For this review, use the dimensioned drawing (mm, ordinates from the lowest corner) and the shaded views. Give positions to 0.01 mm unless a question says otherwise; leave off trailing zeros. Order: outer loops, then holes, each group sorted by start corner. A loop starts at its lowest first (then second) coordinate and runs counter-clockwise, first axis right, second up. Notation, with made-up numbers: (-36, 60) -> (-10, 60) arc R30 cw to (-10, 98) -> close; hole circle Ø7 at (5.5, 52). An arc over 180 degrees is marked (long way). One line per item, written item: value. Start each with the question number.
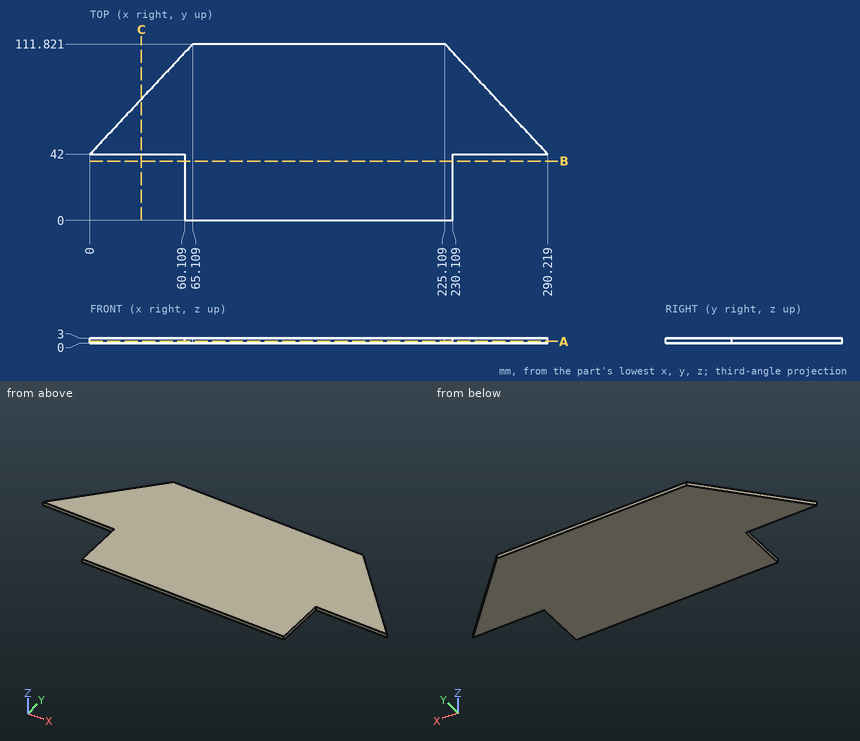
Q1. Take a section at C-C (x = 32.5). State the section outline as (y, z) points, and give its area (3 significant figures).
Q2. Take a section at A-A (z = 1.15). State the section outline as (x, y) points, and give its area (3 significant figures).
Q3. Take a section at B-B (y = 37.5). State the section outline as (x, z) points, and give its area (3 significant figures).
Q4. For line 1 along X through (y, z) = (37, 1.85); line 2 along X through (y, z) = (50.5, 1.7) (1 decimal); line 3 along Y through (x, z) = (272.5, 2), list the stretches that pass through material, from the lowest coordinate up.
Q5. For pin 1 Ø1.5 at (y, z) = (16, 2) entering from +X; pin 2 Ø1.5 at (x, z) = (40, 2) entering from -Y; pin 3 Ø1 at (y, z) = (73, 1.5) entering from -X; pin 4 Ø1.5 at (x, y) = (112, 12.5) entering from -Z, all flat-tipped, find the tip position at first contact; note any pin that passes through.
Answers below:
1. outline: (42, 0) -> (76.85, 0) -> (76.85, 3) -> (42, 3) -> close
1. area: 105 mm²
2. outline: (0, 42) -> (60.11, 42) -> (60.11, 0) -> (230.11, 0) -> (230.11, 42) -> (290.22, 42) -> (225.11, 111.82) -> (65.11, 111.82) -> close
2. area: 22,900 mm²
3. outline: (60.11, 0) -> (230.11, 0) -> (230.11, 3) -> (60.11, 3) -> close
3. area: 510 mm²
4. line 1: x = 60.11 to 230.11
4. line 2: x = 7.9 to 282.3
4. line 3: y = 42 to 61
5. pin 1: stops at x = 230.11
5. pin 2: stops at y = 42
5. pin 3: stops at x = 28.44
5. pin 4: stops at z = 0
